Autodesk Fusion 360 part; units mm, degrees
sketch "Sketch1" plane through (0, 0, 0) normal (0, 0, 1) x (1, 0, 0)
  line L0 (20, 20) -> (-20, 20)
  line L1 (-20, 20) -> (-20, -20)
  line L2 (-20, -20) -> (20, -20)
  line L3 (20, -20) -> (20, 20)
  line L4 (20, 20) -> (-20, -20) construction
  line L5 (-20, 20) -> (20, -20) construction
  circle A0 centre (0, 0) radius 10
  line L6 (13, -13) -> (-13, -13) construction
  line L7 (-13, -13) -> (-13, 13) construction
  line L8 (-13, 13) -> (13, 13) construction
  line L9 (13, 13) -> (13, -13) construction
  line L10 (13, -13) -> (-13, 13) construction
  line L11 (-13, -13) -> (13, 13) construction
  circle A1 centre (-13, 13) radius 2
  circle A2 centre (13, 13) radius 2
  circle A3 centre (13, -13) radius 2
  circle A4 centre (-13, -13) radius 2
  dimension "d1" = 40
  dimension "d2" = 40
  dimension "d3" = 20
  dimension "d6" = 26
  dimension "d7" = 26
  dimension "d8" = 4
  dimension "d9" = 4
  dimension "d10" = 4
  dimension "d11" = 4
extrude "Extrude1" add sketch "Sketch1" along normal blind 9
chamfer "Chamfer1" distance 2.5 angle 45 4 edges at (-14.8647, 13.7232, 9) (-14.8647, -12.2768, 9) (11.1353, -12.2768, 9) (11.1353, 13.7232, 9)
equation "d9 = d8"
equation "d10 = d8"
equation "d11 = d8"
Verification items for the finished model (mm, model axes). Coordinates: 2 decimals unless noted, no trailing zeros. Order: outer loops, then holes, each group sorted by start corner. A loop starts at its lowest first (then second) coordinate and runs counter-clockwise, first axis right, second up.
1. Sectioned sample at B-B, the plane y = -13. Record the cut outline in (x, z), and give its area (4 significant figures).
Results found:
outline: (-20, 0) - (-15, 0) - (-15, 6.5) - (-17.5, 9) - (-20, 9) - close; (-11, 0) - (11, 0) - (11, 6.5) - (8.5, 9) - (-8.5, 9) - (-11, 6.5) - close; (15, 0) - (20, 0) - (20, 9) - (17.5, 9) - (15, 6.5) - close
area: 275.5 mm2
2. Sectioned sample at A-A, the plane z = 7. Record the cut outline in (x, y).
Results found:
outline: (-20, -20) - (20, -20) - (20, 20) - (-20, 20) - close; hole circle Ø5 at (-13, -13); hole circle Ø5 at (-13, 13); hole circle Ø20 at (0, 0); hole circle Ø5 at (13, -13); hole circle Ø5 at (13, 13)
3. Release check for a two-part mould opening along X. For faces 1 (the face through (0, -20, 4)), 2 (the face through (-20, 0, 4)), 3 (the face through (14.16, -11.18, 6.66)) record: +X half, -X half, draft (parallel to the pull), parting line (faces both ways), or undercut.
Results found:
face 1: draft
face 2: -X half
face 3: undercut
4. Go/stop test with flat-tipped pins: pin 1 Ø6.5 at (x, y) = (13, -13) entering from +Z; pin 2 Ø3 at (x, y) = (-13, -13) entering from -Z; pin 3 Ø8 at (x, y) = (6.5, -2.5) entering from -Z. Record where each tip stops, or that it passes through.
Results found:
pin 1: stops at z = 7.75
pin 2: passes through
pin 3: stops at z = 0
5. Scan lines: line 1 (Y direction, x = -13, z = 2.25); line 2 (Y direction, x = 0, z = 4.75); line 3 (Y direction, x = -14, z = 6.5). Record each from-to range of solid material in increasing order.
Results found:
line 1: y = -20 to -15, -11 to 11, 15 to 20
line 2: y = -20 to -10, 10 to 20
line 3: y = -20 to -14.73, -11.27 to 11.27, 14.73 to 20
6. Sectioned sample at C-C, the plane x = 0. Record the cut outline in (y, z), and give its area (3 significant figures).
Results found:
outline: (-20, 0) - (-10, 0) - (-10, 9) - (-20, 9) - close; (10, 0) - (20, 0) - (20, 9) - (10, 9) - close
area: 180 mm2
